```python
from build123d import *

# Parameters (mm, degrees)
SKETCH1_R           = 8.73125
BOSS_EXTRUDE1_DEPTH = 11
CUT_EXTRUDE1_DEPTH  = 17.536911838
CIRPATTERN1_COUNT   = 20
SKETCH4_R           = 2.5
CUT_EXTRUDE2_DEPTH  = 3.3
SKETCH5_R           = 1
CUT_EXTRUDE3_DEPTH  = 15.465788277


with BuildPart() as part:
    # Sketch1 → Boss-Extrude1 (new body)
    with BuildSketch(Plane.XY):
        Circle(SKETCH1_R)
    extrude(amount=BOSS_EXTRUDE1_DEPTH)

    # Sketch2 → Cut-Extrude1 (cut, through all)
    with BuildSketch(Plane.XY.offset(11)):
        with BuildLine():
            Line((9.170880897, -1.77931535), (9.170880897, 1.77931535))
            ThreePointArc((9.170880897, 1.77931535), (8.236219229, 0.806271061), (6.929309614, 0.4710176))
            ThreePointArc((6.929309614, 0.4710176), (6.9452998, 0), (6.929309614, -0.4710176))
            ThreePointArc((6.929309614, -0.4710176), (8.236219229, -0.806271061), (9.170880897, -1.77931535))
        make_face()
    cut_extrude1 = extrude(amount=-CUT_EXTRUDE1_DEPTH, mode=Mode.SUBTRACT)

    # CirPattern1: Cut-Extrude1 ×20 about axis
    cirpattern1_axis = Axis((0, 0, 0), (0, 0, 1))
    for i in range(1, CIRPATTERN1_COUNT):
        add(cut_extrude1.rotate(cirpattern1_axis, i * 360 / CIRPATTERN1_COUNT), mode=Mode.SUBTRACT)

    # Sketch4 → Cut-Extrude2 (cut)
    with BuildSketch(Plane.XY.offset(11)):
        Circle(SKETCH4_R)
    extrude(amount=-CUT_EXTRUDE2_DEPTH, mode=Mode.SUBTRACT)

    # Sketch5 → Cut-Extrude3 (cut, through all)
    with BuildSketch(Plane.XY.offset(7.7)):
        Circle(SKETCH5_R)
    extrude(amount=-CUT_EXTRUDE3_DEPTH, mode=Mode.SUBTRACT)


solid = part.part
```
Could you check a few things on this model? Use its own coordinates, in mm. A direction names the side the tool comes from. Round coordinates to 2 decimals unless told otherwise and drop trailing zeros. Loops run counter-clockwise (first coordinate to the right, second up) from the corner with the lowest first, then second, coordinate; pieces in that order, holes last. Notation, with made-up numbers: (5, -37.5) -> (31, -37.5) arc R24 ccw to (31, -7.5) -> close; hole circle Ø4 at (55, 71.25). An arc over 180 degrees is marked (long way). Put each result on its own line as item: value.
Q1. I want a section at D-D on y = -5. Write out the boundary of the cut face in (x, z).
Checks:
outline: (-5.9, 0) -> (5.9, 0) -> (5.9, 11) -> (-5.9, 11) -> close
Q2. I want a section at A-A on y = 0. Write out the boundary of the cut face in (x, z).
Checks:
outline: (-6.95, 0) -> (-1, 0) -> (-1, 7.7) -> (-2.5, 7.7) -> (-2.5, 11) -> (-6.95, 11) -> close; (1, 0) -> (6.95, 0) -> (6.95, 11) -> (2.5, 11) -> (2.5, 7.7) -> (1, 7.7) -> close
Q3. Which directions (+Z, -Z, +X, -X, +Y, -Y) give clear straight access to the entire face, cutting with the end or side of a thin tool? Please do faces 3 (the cylindrical face through (6.945, 0.007, 5.577)), 4 (the cylindrical face through (-7.653, -1.833, 5.577)).
Checks:
face 3: +Z, -Z, +X
face 4: +Z, -Z
Q4. Thinking about a two-plate mould opening in X: for faces 1 (the cylindrical face through (5.98, -5.11, 5.58)), 2 (the cylindrical face through (6.712, 4.108, 5.577)), which applies, pulls with the +X half, pulls with the -X half, needs draft (parallel to the pull), parting line crosses it, or undercut?
Checks:
face 1: pulls with the +X half
face 2: undercut
Q5. Please list where these lines run through material, in increasing order: line 1 (Y direction, x = -5.75, z = 10.5); line 2 (Y direction, x = 0, z = 5); line 3 (Y direction, x = 0, z = 8.4). Write a range as from..to.
Checks:
line 1: -6.29..-4.82, -3.9..3.9, 4.82..6.29
line 2: -6.95..-1, 1..6.95
line 3: -6.95..-2.5, 2.5..6.95
Q6. I want a section at C-C on x = -7.25. Write out the boundary of the cut face in (y, z), and give its area (3 significant figures).
Checks:
outline: (-4.2, 0) -> (-3, 0) -> (-3, 11) -> (-4.2, 11) -> close; (-1.82, 0) -> (-0.48, 0) -> (-0.48, 11) -> (-1.82, 11) -> close; (0.48, 0) -> (1.82, 0) -> (1.82, 11) -> (0.48, 11) -> close; (3, 0) -> (4.2, 0) -> (4.2, 11) -> (3, 11) -> close
area: 55.6 mm2
Q7. For pin 1 Ø2 at (x, y) = (3, -2.5) entering from -Z; pin 2 Ø4 at (x, y) = (0, 0) entering from +Z; pin 3 Ø1.6 at (x, y) = (0, 0) entering from +Z (3 decimals); pin 4 Ø1.5 at (y, z) = (3.5, 9.5) entering from +X, each with a flat end and sliding along its axis, tell me the tip position at first contact or that it passes through.
Checks:
pin 1: z = 0
pin 2: z = 7.7
pin 3: through
pin 4: x = 7.89
